```python
from build123d import *

# Parameters (mm, degrees)
SKETCH1_R               = 24.257
SKETCH1_R_2             = 19.05
BOSS_EXTRUDE1_DEPTH     = 114.3
CUT_EXTRUDE1_DEPTH      = 120.336893281
CUT_EXTRUDE1_DEPTH_BACK = 2.54
SKETCH2_W               = 30.48
SKETCH2_H               = 63.5


with BuildPart() as part:
    # Sketch1 → Boss-Extrude1 (new body)
    with BuildSketch(Plane.XY):
        Circle(SKETCH1_R)
        Circle(SKETCH1_R_2, mode=Mode.SUBTRACT)
    extrude(amount=BOSS_EXTRUDE1_DEPTH)

    # Sketch2 → Cut-Extrude1 (cut, two sides: drawn at the far end of the back side and taken through both)
    with BuildSketch(Plane(origin=(0, 0, 0), x_dir=(1, 0, 0), z_dir=(0, 1, 0)).offset(-CUT_EXTRUDE1_DEPTH_BACK)):
        with Locations((0, -31.75)):
            Rectangle(SKETCH2_W, SKETCH2_H)
    extrude(amount=CUT_EXTRUDE1_DEPTH + CUT_EXTRUDE1_DEPTH_BACK, mode=Mode.SUBTRACT)


solid = part.part
```
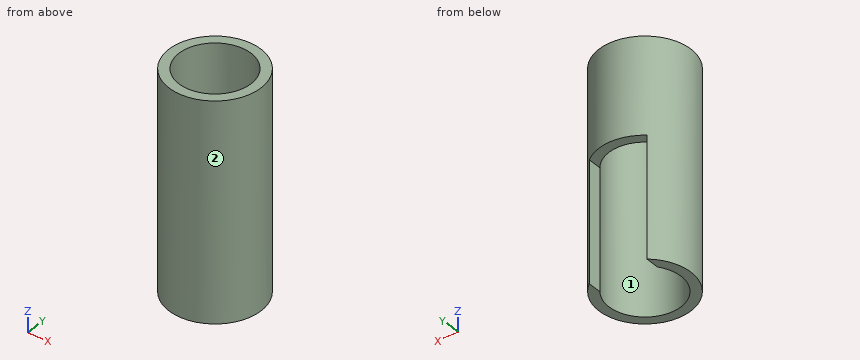
Here's how the part is built. I have some questions about the finished solid (model axes, mm). Face numbers are marked on the shaded views. Round coordinates to 2 decimals unless told otherwise and drop trailing zeros. Order: outer loops, then holes, each group sorted by start corner. A loop starts at its lowest first (then second) coordinate and runs counter-clockwise, first axis right, second up. Notation, with made-up numbers: M 55,31 L 67,31 A23 ccw 67,67 Z; hole C 26.25,-9.75 d2. An arc over 180 degrees is marked long. Answer in a Markdown table with one row per item.
Item 1: Imagine slicing it at D-D, the plane y = 13. Write out the boundary of the cut face in (x, z).
A:
| item | result |
|---|---|
| outline | M -20.48,0 L -15.24,0 L -15.24,63.5 L -13.92,63.5 L -13.92,114.3 L -20.48,114.3 Z; M 13.92,63.5 L 15.24,63.5 L 15.24,0 L 20.48,0 L 20.48,114.3 L 13.92,114.3 Z |
Item 2: If I drill on L1, parallel to X at y = 0, z = 65.5; L2, parallel to Z at x = -10.5, y = 19.5; L3, parallel to Y at x = -14, z = 108, over which ranges is the centre line in solid material (lowest first)? Write a range as from..to.
A:
| item | result |
|---|---|
| L1 | x = -24.26..-19.05, 19.05..24.26 |
| L2 | z = 63.5..114.3 |
| L3 | y = -19.81..-12.92, 12.92..19.81 |
Item 3: Imagine slicing it at A-A, the plane y = 0. Write out the boundary of the cut face in (x, z), and give its area (3 significant figures).
A:
| item | result |
|---|---|
| outline | M -24.26,0 L -19.05,0 L -19.05,114.3 L -24.26,114.3 Z; M 19.05,0 L 24.26,0 L 24.26,114.3 L 19.05,114.3 Z |
| area | 1,190 mm2 |
Item 4: Imagine slicing it at C-C, the plane z = 80. Write out the boundary of the cut face in (x, y), and give its area (3 significant figures).
A:
| item | result |
|---|---|
| outline | C 0,0 d48.51; hole C 0,0 d38.1 |
| area | 708 mm2 |
Item 5: Imagine slicing it at B-B, the plane x = 0. Write out the boundary of the cut face in (y, z).
A:
| item | result |
|---|---|
| outline | M -24.26,0 L -19.05,0 L -19.05,114.3 L -24.26,114.3 Z; M 19.05,63.5 L 24.26,63.5 L 24.26,114.3 L 19.05,114.3 Z |
Item 6: Thinking about a two-plate mould opening in Y: for the marked faces 1 and 2, which applies, +Y half, -Y half, draft (parallel to the pull), parting line (faces both ways), or undercut?
A:
| item | result |
|---|---|
| face 1 | undercut |
| face 2 | parting line |
Item 7: I'm going to push flat-ended pins straight in: pin 1 (2 mm diameter, centred on y = 15.5, z = 18.5, fed in from -X); pin 2 (1 mm diameter, centred on y = 9.5, z = 49, fed in from -X); pin 3 (2 mm diameter, centred on y = 14, z = 19.5, fed in from +X); pin 4 (2 mm diameter, centred on x = -17, y = -1, fed in from +Z). Where does each tip first touch, or does it pass through?
A:
| item | result |
|---|---|
| pin 1 | stops at x = -19.45 |
| pin 2 | stops at x = -22.53 |
| pin 3 | stops at x = 20.48 |
| pin 4 | passes through |
